from build123d import *

# Parameters (mm, degrees)
RIB1_REACH              = 112.498
SKETCH2_WALL_W          = 261.642553204
SKETCH2_WALL_H          = 6
CUT_EXTRUDE2_DEPTH      = 111.497997453
CUT_EXTRUDE2_DEPTH_BACK = 10
SKETCH4_R               = 7.5
CIRPATTERN6_COUNT       = 4


with BuildPart() as part:
    # Sketch1 → Revolve1 (revolve)
    with BuildSketch(Plane.XY, mode=Mode.PRIVATE) as revolve1_sk:
        Polygon((20, 49.089789582), (20, -0.910210418), (70, -0.910210418), (70, 14.089789582), (40, 14.089789582), (40, 49.089789582), align=None)
    revolve(revolve1_sk.sketch.rotate(Axis((0, 0, 0), (0, 1, 0)), 90), axis=Axis((0, 0, 0), (0, 1, 0)))

    # Sketch2 wall → Rib1 (add, up to next)
    with BuildSketch(Plane(origin=(-52.5, 29.354148536, 0), x_dir=(0.646888134458, 0.76258490773, 0), z_dir=(-0.76258490773, 0.646888134458, 0)), mode=Mode.PRIVATE) as rib1_sk1:
        Rectangle(SKETCH2_WALL_W, SKETCH2_WALL_H)
    rib1_tool1 = extrude(rib1_sk1.sketch, amount=-RIB1_REACH, mode=Mode.PRIVATE) - part.part
    rib1 = rib1_tool1.solids().sort_by_distance((-52.5, 29.354148536, 0))[0]
    add(rib1)

    # Sketch4 → Cut-Extrude2 (cut, two sides: drawn at the far end of the back side and taken through both)
    with BuildSketch(Plane(origin=(0, 0, 0), x_dir=(1, 0, 0), z_dir=(0, 1, 0)).offset(-CUT_EXTRUDE2_DEPTH_BACK)):
        with Locations(Location((-39.62662351, 38.140932201, 0), (0, 0, 270))):
            Circle(SKETCH4_R)
        with Locations(Location((38.140932201, 39.62662351, 0), (0, 0, 270))):
            Circle(SKETCH4_R)
        with Locations(Location((39.62662351, -38.140932201, 0), (0, 0, 270))):
            Circle(SKETCH4_R)
        with Locations(Location((-38.140932201, -39.62662351, 0), (0, 0, 270))):
            Circle(SKETCH4_R)
    extrude(amount=CUT_EXTRUDE2_DEPTH + CUT_EXTRUDE2_DEPTH_BACK, mode=Mode.SUBTRACT)

    # CirPattern6: Rib1 ×4 about axis
    cirpattern6_axis = Axis((0, 0, 0), (0, 1, 0))
    for i in range(1, CIRPATTERN6_COUNT):
        add(rib1.rotate(cirpattern6_axis, i * 360 / CIRPATTERN6_COUNT))


solid = part.part
CAD build for the part. Positions are in the model's coordinates, mm. A direction names the side the tool comes from. Give positions to 0.01 mm unless a question says otherwise; leave off trailing zeros. Order: outer loops, then holes, each group sorted by start corner. A loop starts at its lowest first (then second) coordinate and runs counter-clockwise, first axis right, second up. Notation, with made-up numbers: (70.5, 58) - (112.5, 58) arc R17 ccw to (112.5, 71) - close; hole circle Ø5 at (24, -9). An arc over 180 degrees is marked (long way). Answer in a Markdown table with one row per item.
1. Saw through at B-B, the plane y = 38.5. Give the cut face in (x, z).
Data:
| item | result |
|---|---|
| outline | (-44.74, -3) - (-39.89, -3) arc R40 ccw to (-3, -39.89) - (-3, -44.74) - (3, -44.74) - (3, -39.89) arc R40 ccw to (39.89, -3) - (44.74, -3) - (44.74, 3) - (39.89, 3) arc R40 ccw to (3, 39.89) - (3, 44.74) - (-3, 44.74) - (-3, 39.89) arc R40 ccw to (-39.89, 3) - (-44.74, 3) - close; hole circle Ø40 at (0, 0) |
2. Tool access for faces 4 (the flat face through (3, 26, -49)), 5 (the flat face through (-3, 26, 49)), 6 (the flat face through (-49, 26, -3)): list every direction of +Z, -Z, +X, -X, +Y, -Y with a clear straight run to the whole face (end or side of a thin tool).
Data:
| item | result |
|---|---|
| face 4 | -Z, +X, +Y |
| face 5 | +Z, -X, +Y |
| face 6 | -Z, -X, +Y |
3. Saw through at C-C, the plane z = 42. Give the cut face in (x, y).
Data:
| item | result |
|---|---|
| outline | (-56, -0.91) - (-45.26, -0.91) - (-45.26, 14.09) - (-56, 14.09) - close; (-31.03, -0.91) - (33.2, -0.91) - (33.2, 14.09) - (3, 14.09) - (3, 41.73) - (-3, 41.73) - (-3, 14.09) - (-31.03, 14.09) - close; (46.06, -0.91) - (56, -0.91) - (56, 14.09) - (46.06, 14.09) - close |
4. Saw through at A-A, the plane x = 0. Give the cut face in (y, z).
Data:
| item | result |
|---|---|
| outline | (-0.91, -70) - (14.09, -70) - (14.09, -65.45) - (44.09, -40) - (49.09, -40) - (49.09, -20) - (-0.91, -20) - close; (-0.91, 20) - (49.09, 20) - (49.09, 40) - (44.09, 40) - (14.09, 65.45) - (14.09, 70) - (-0.91, 70) - close |
5. Flat gauge pins, fed straight in: pin 1 (12 mm diameter, centred on x = 22.5, y = 7.5, fed in from -Z); pin 2 (7.5 mm diameter, centred on y = 31.5, z = 51.5, fed in from -X); pin 3 (17 mm diameter, centred on x = 38.14, z = -39.63, fed in from +Y); pin 4 (12 mm diameter, centred on x = 39.63, z = 38.14, fed in from -Y). Where does each tip first touch, or does it go through?
Data:
| item | result |
|---|---|
| pin 1 | stops at z = -68.03 |
| pin 2 | stops at x = -3 |
| pin 3 | stops at y = 14.09 |
| pin 4 | passes through |
6. Pull direction X, two halves, no side cores. Call faces 1 (the flat face through (-49, 26, 3)), 2 (the cylindrical face through (39.96, 6.48, 30.65)), 3 (the flat face through (52.847, 28.945, 0.042)): pulls with the +X half, pulls with the -X half, needs draft (parallel to the pull), parting line crosses it, or undercut.
Data:
| item | result |
|---|---|
| face 1 | needs draft |
| face 2 | undercut |
| face 3 | pulls with the +X half |
7. Saw through at D-D, the plane z = -13. Give the cut face in (x, y).
Data:
| item | result |
|---|---|
| outline | (-68.78, -0.91) - (-15.2, -0.91) - (-15.2, 49.09) - (-37.83, 49.09) - (-37.83, 14.09) - (-68.78, 14.09) - close; (15.2, -0.91) - (68.78, -0.91) - (68.78, 14.09) - (37.83, 14.09) - (37.83, 49.09) - (15.2, 49.09) - close |
8. Probe probe 1 along Y at (x, z) = (16, -40); probe 2 along Z at (x, y) = (0.5, 42.5); probe 3 along X at (y, z) = (20, 0). List the from-to ranges inside material, lowest first. Write a range as [from, to].
Data:
| item | result |
|---|---|
| probe 1 | y = [-0.91, 14.09] |
| probe 2 | z = [-41.35, -19.99], [19.99, 41.35] |
| probe 3 | x = [-60.43, -20], [20, 60.43] |
